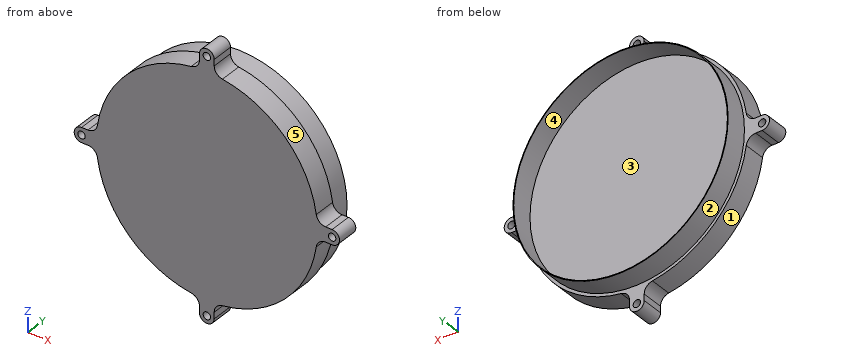
```python
from build123d import *

# Parameters (mm, degrees)
SKETCH2_R           = 146
SKETCH2_R_2         = 145
BOSS_EXTRUDE2_DEPTH = 30
SKETCH3_R           = 5
BOSS_EXTRUDE4_DEPTH = 30


with BuildPart() as part:
    # Sketch2 → Boss-Extrude2 (new body)
    with BuildSketch(Plane(origin=(0, 0, 0), x_dir=(1, 0, 0), z_dir=(0, 1, 0))):
        Circle(SKETCH2_R)
        Circle(SKETCH2_R_2, mode=Mode.SUBTRACT)
    extrude(amount=BOSS_EXTRUDE2_DEPTH)

    # Sketch3 → Boss-Extrude4 (add)
    with BuildSketch(Plane(origin=(0, 0, 0), x_dir=(1, 0, 0), z_dir=(0, 1, 0))):
        with BuildLine():
            Line((161.369142032, 10), (170, 10))
            ThreePointArc((170, 10), (180, 0), (170, -10))
            Line((170, -10), (161.369142032, -10))
            ThreePointArc((161.369142032, -10), (152.849946816, -13.180462695), (148.499210458, -21.165644172))
            ThreePointArc((148.499210458, -21.165644172), (106.066017178, -106.066017178), (21.165644172, -148.499210458))
            ThreePointArc((21.165644172, -148.499210458), (13.180462695, -152.849946816), (10, -161.369142032))
            Line((10, -161.369142032), (10, -170))
            ThreePointArc((10, -170), (0, -180), (-10, -170))
            Line((-10, -170), (-10, -161.369142032))
            ThreePointArc((-10, -161.369142032), (-13.180462695, -152.849946816), (-21.165644172, -148.499210458))
            ThreePointArc((-21.165644172, -148.499210458), (-106.066017178, -106.066017178), (-148.499210458, -21.165644172))
            ThreePointArc((-148.499210458, -21.165644172), (-152.849946816, -13.180462695), (-161.369142032, -10))
            Line((-161.369142032, -10), (-170, -10))
            ThreePointArc((-170, -10), (-180, 0), (-170, 10))
            Line((-170, 10), (-161.369142032, 10))
            ThreePointArc((-161.369142032, 10), (-152.849946816, 13.180462695), (-148.499210458, 21.165644172))
            ThreePointArc((-148.499210458, 21.165644172), (-106.066017178, 106.066017178), (-21.165644172, 148.499210458))
            ThreePointArc((-21.165644172, 148.499210458), (-13.180462695, 152.849946816), (-10, 161.369142032))
            Line((-10, 161.369142032), (-10, 170))
            ThreePointArc((-10, 170), (0, 180), (10, 170))
            Line((10, 170), (10, 161.369142032))
            ThreePointArc((10, 161.369142032), (13.180462695, 152.849946816), (21.165644172, 148.499210458))
            ThreePointArc((21.165644172, 148.499210458), (106.066017178, 106.066017178), (148.499210458, 21.165644172))
            ThreePointArc((148.499210458, 21.165644172), (152.849946816, 13.180462695), (161.369142032, 10))
        make_face()
        with Locations((0, 170)):
            Circle(SKETCH3_R, mode=Mode.SUBTRACT)
        with Locations((170, 0)):
            Circle(SKETCH3_R, mode=Mode.SUBTRACT)
        with Locations((0, -170)):
            Circle(SKETCH3_R, mode=Mode.SUBTRACT)
        with Locations((-170, 0)):
            Circle(SKETCH3_R, mode=Mode.SUBTRACT)
    extrude(amount=-BOSS_EXTRUDE4_DEPTH)


solid = part.part
```
Geometry: final body of the model. Coordinates: model frame, mm. Face numbers are marked on the shaded views. A direction names the side the tool comes from. Give positions to 0.01 mm unless a question says otherwise; leave off trailing zeros. Loops run counter-clockwise (first coordinate to the right, second up) from the corner with the lowest first, then second, coordinate; pieces in that order, holes last. Notation, with made-up numbers: (63.5, -26.75) -> (113.5, -26.75) arc R25 cw to (113.5, -2.75) -> close; hole circle Ø8 at (81.25, -40). An arc over 180 degrees is marked (long way). Use one line per item in the form item = value.
Item 1: Section query A-A on z = 0. Output: boundary loops of the cut face in (x, y), and give its area (3 significant figures).
A:
outline = (-180, -30) -> (-175, -30) -> (-175, 0) -> (-180, 0) -> close; (-165, -30) -> (165, -30) -> (165, 0) -> (146, 0) -> (146, 30) -> (145, 30) -> (145, 0) -> (-145, 0) -> (-145, 30) -> (-146, 30) -> (-146, 0) -> (-165, 0) -> close; (175, -30) -> (180, -30) -> (180, 0) -> (175, 0) -> close
area = 10,300 mm^2
Item 2: Section query D-D on z = 68. Output: boundary loops of the cut face in (x, y).
A:
outline = (-133.7, -30) -> (133.7, -30) -> (133.7, 0) -> (129.2, 0) -> (129.2, 30) -> (128.07, 30) -> (128.07, 0) -> (-128.07, 0) -> (-128.07, 30) -> (-129.2, 30) -> (-129.2, 0) -> (-133.7, 0) -> close
Item 3: Draft query along X for the marked faces 1, 2 and 3. Return one class per face: pulls with the +X half, pulls with the -X half, needs draft (parallel to the pull), parting line crosses it, or undercut.
A:
face_1 = pulls with the -X half
face_2 = parting line crosses it
face_3 = undercut
Item 4: Access query for the marked faces 4 and 5. Directions: +Z, -Z, +X, -X, +Y, -Y. A direction counts if a zero-diameter tool reaches every point of the face in a straight line with its end or side. Return the directions, or none.
A:
face_4 = +Y
face_5 = +Z, +X, +Y, -Y
Item 5: Section query C-C on y = -15. Output: boundary loops of the cut face in (x, z).
A:
outline = (-170, -10) -> (-161.37, -10) arc R13 cw to (-148.5, -21.17) arc R150 ccw to (-21.17, -148.5) arc R13 cw to (-10, -161.37) -> (-10, -170) arc R10 ccw to (10, -170) -> (10, -161.37) arc R13 cw to (21.17, -148.5) arc R150 ccw to (148.5, -21.17) arc R13 cw to (161.37, -10) -> (170, -10) arc R10 ccw to (170, 10) -> (161.37, 10) arc R13 cw to (148.5, 21.17) arc R150 ccw to (21.17, 148.5) arc R13 cw to (10, 161.37) -> (10, 170) arc R10 ccw to (-10, 170) -> (-10, 161.37) arc R13 cw to (-21.17, 148.5) arc R150 ccw to (-148.5, 21.17) arc R13 cw to (-161.37, 10) -> (-170, 10) arc R10 ccw to start; hole circle Ø10 at (-170, 0); hole circle Ø10 at (0, -170); hole circle Ø10 at (0, 170); hole circle Ø10 at (170, 0)
Item 6: Line query: probe 1 along X at (y, z) = (-15.75, 0); probe 2 along X at (y, z) = (-9, -170). Output: solid intervals per line, ascending.
A:
probe_1 = -180 to -175, -165 to 165, 175 to 180
probe_2 = -10 to -5, 5 to 10
Item 7: Pin query (flat end, axial travel): P1, Ø10, axis at y = 10, z = -83.5, coming from the +X side; P2, Ø4.5, axis at x = 165.5, y = -19.5, coming from the +Z side; P3, Ø13, axis at x = 170, z = 0, coming from the +Y side. Return the tip coordinate at first contact, or that it passes through.
A:
P1 = 123.1
P2 = 10
P3 = 0
Item 8: Section query B-B on x = 0. Output: boundary loops of the cut face in (y, z).
A:
outline = (-30, -180) -> (0, -180) -> (0, -175) -> (-30, -175) -> close; (-30, -165) -> (0, -165) -> (0, -146) -> (30, -146) -> (30, -145) -> (0, -145) -> (0, 145) -> (30, 145) -> (30, 146) -> (0, 146) -> (0, 165) -> (-30, 165) -> close; (-30, 175) -> (0, 175) -> (0, 180) -> (-30, 180) -> close
